from build123d import *

# Parameters (mm, degrees)
EXTRUDE064_DEPTH           = 5
EXTRUDE066_DEPTH           = 5
EXTRUDE066_PLACEMENT_ANGLE = 180
EXTRUDE065_DEPTH           = 2
EXTRUDE065_PLACEMENT_ANGLE = 180
EXTRUDE061_DEPTH           = 2
EXTRUDE063_DEPTH           = 3
EXTRUDE060_DEPTH           = 10
EXTRUDE057_DEPTH           = 5


with BuildPart() as extrude064:
    # Sketch039 → Extrude064 (new body)
    with BuildSketch(Plane.XY):
        Polygon((-0.523418, -66.073971), (-3.588769, -58.006004), (-3.588769, -66.073971), align=None)
    extrude(amount=EXTRUDE064_DEPTH)


with BuildPart() as extrude064_1:
    # Extrude064 placement: moved
    add(extrude064.part.moved(Location((-2, 0, -1))))


with BuildPart() as fusion056:
    # Sketch039 → Extrude066 (new body)
    with BuildSketch(Plane.XY):
        Polygon((-0.523418, -66.073971), (-3.588769, -58.006004), (-3.588769, -66.073971), align=None)
    extrude(amount=EXTRUDE066_DEPTH)


with BuildPart() as fusion056_1:
    # Extrude066 placement: moved
    add(fusion056.part.moved(Location((-2, -63.2, 3.5))).rotate(Axis((-2, -63.2, 3.5), (1, 0, 0)), EXTRUDE066_PLACEMENT_ANGLE))

    # Fusion056: union Extrude064
    add(extrude064_1.part)


with BuildPart() as extrude065:
    # Sketch037 → Extrude065 (new body)
    with BuildSketch(Plane.XY):
        Polygon((-0.523418, -66.073971), (-3.588769, -58.006004), (-3.588769, -66.073971), align=None)
    extrude(amount=EXTRUDE065_DEPTH)


with BuildPart() as extrude065_1:
    # Extrude065 placement: moved
    add(extrude065.part.moved(Location((-0.5, -63.2, 2.45))).rotate(Axis((-0.5, -63.2, 2.45), (1, 0, 0)), EXTRUDE065_PLACEMENT_ANGLE))


with BuildPart() as fusion055:
    # Sketch037 → Extrude061 (new body)
    with BuildSketch(Plane.XY):
        Polygon((-0.523418, -66.073971), (-3.588769, -58.006004), (-3.588769, -66.073971), align=None)
    extrude(amount=EXTRUDE061_DEPTH)


with BuildPart() as fusion055_1:
    # Extrude061 placement: moved
    add(fusion055.part.moved(Location((-0.5, 0, 0.4))))

    # Fusion055: union Extrude065
    add(extrude065_1.part)


with BuildPart() as extrude063:
    # Sketch038 → Extrude063 (new body)
    with BuildSketch(Plane.YZ):
        with BuildLine():
            ThreePointArc((-52.009312, -0.734582), (-31.50638, -4.580156), (-11.018523, -0.655055))
            ThreePointArc((-5.240026, 0.419738), (-8.178332, 0.146093), (-11.018523, -0.655055))
            Line((-5.240026, 0.419738), (2.759974, 0.419738))
            Line((2.759974, 0.419738), (2.759974, 2.419738))
            Line((2.759974, 2.419738), (-5.240026, 2.419738))
            ThreePointArc((-5.240026, 2.419738), (-8.772288, 2.061286), (-12.172965, 1.041109))
            ThreePointArc((-51.872542, 1.363439), (-32.05345, -2.578482), (-12.172965, 1.041109))
            ThreePointArc((-51.872542, 1.363439), (-54.88716, 2.147131), (-57.990026, 2.419738))
            Line((-65.990026, 2.419738), (-57.990026, 2.419738))
            Line((-65.990026, 0.419738), (-65.990026, 2.419738))
            Line((-57.990026, 0.419738), (-65.990026, 0.419738))
            ThreePointArc((-52.009312, -0.734582), (-54.946975, 0.115595), (-57.990026, 0.419738))
        make_face()
    extrude(amount=EXTRUDE063_DEPTH)


with BuildPart() as extrude063_1:
    # Extrude063 placement: moved
    add(extrude063.part.moved(Location((-7, 0, 0))))


with BuildPart() as extrude060:
    # Sketch036 → Extrude060 (new body)
    with BuildSketch(Plane.XY):
        Polygon((-0.489114, -59.765606), (-2.785057, -58.065606), (-2.989114, -56.006916), (-2.989114, -7.606139), (-2.772346, -5.215606), (-0.489114, -3.515606), align=None)
    extrude(amount=EXTRUDE060_DEPTH)


with BuildPart() as extrude060_1:
    # Extrude060 placement: moved
    add(extrude060.part.moved(Location((0, 0, -6))))


with BuildPart() as obj1:
    # Sketch033 → Extrude057 (new body)
    with BuildSketch(Plane.YZ):
        with BuildLine():
            ThreePointArc((-52.506138, -1.600172), (-31.607264, -5.496793), (-10.720935, -1.533483))
            ThreePointArc((-5.324033, -0.496866), (-8.066716, -0.784889), (-10.720935, -1.533483))
            Line((-5.324033, -0.496866), (2.675967, -0.496866))
            Line((2.675967, -0.496866), (2.675967, 3.003134))
            Line((2.675967, 3.003134), (-5.324033, 3.003134))
            ThreePointArc((-5.324033, 3.003134), (-8.649812, 2.668233), (-11.870907, 1.7752))
            ThreePointArc((-52.088632, 2.000492), (-32.001526, -1.996019), (-11.870907, 1.7752))
            ThreePointArc((-52.088632, 2.000492), (-55.042543, 2.733373), (-58.074033, 3.003134))
            Line((-66.074033, 3.003134), (-58.074033, 3.003134))
            Line((-66.074033, -0.496866), (-66.074033, 3.003134))
            Line((-58.074033, -0.496866), (-66.074033, -0.496866))
            ThreePointArc((-52.506138, -1.600172), (-55.241791, -0.804798), (-58.074033, -0.496866))
        make_face()
    extrude(amount=EXTRUDE057_DEPTH)


with BuildPart() as obj1_1:
    # Extrude057 placement: moved
    add(obj1.part.moved(Location((-5.5, 0.1, 0.15))))

    # Cut060: cut Extrude060
    add(extrude060_1.part, mode=Mode.SUBTRACT)

    # Cut061: cut Extrude063
    add(extrude063_1.part, mode=Mode.SUBTRACT)

    # Cut062: cut Fusion055
    add(fusion055_1.part, mode=Mode.SUBTRACT)

    # Cut063: cut Fusion056
    add(fusion056_1.part, mode=Mode.SUBTRACT)


with BuildPart() as obj1_2:
    # Cut063 placement: moved
    add(obj1_1.part.moved(Location((0, 0, -0.15))))


solid = obj1_2.part
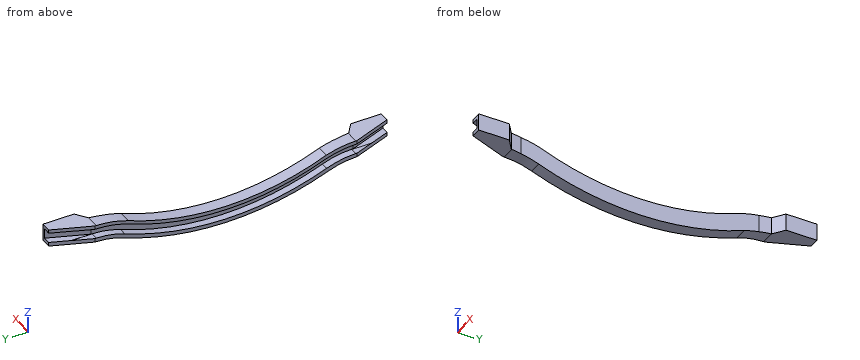
The model under review builds one solid part; all positions refer to its coordinate system, in mm. Coordinates: 2 decimals unless noted, no trailing zeros. Write each loop counter-clockwise with the first axis right and the second up, starting at its lowest first coordinate (ties: lowest second). Pieces come first, ordered by that corner, then holes. Notation, with made-up numbers: M 22.5,-30 L 75.5,-30 A13 cw 75.5,-11 Z; hole C 55,-35.75 d8. An arc over 180 degrees is marked long. Put each result on its own line as item: value.
1) Clearance check with flat-ended pins moving along their axes: pin 1 Ø2 at (x, y) = (-4.5, -44.5) entering from -Z; pin 2 Ø2.5 at (x, y) = (-3.5, -60.5) entering from -Z. State where each tip first meets the part, or that it passes through.
Computed:
pin 1: stops at z = -4.25
pin 2: stops at z = -0.5
2) Add section A-A on y = -33.5. Give the boundary of the cut face in (x, z).
Computed:
outline: M -5.5,-5.47 L -2.99,-5.47 L -2.99,-1.96 L -5.5,-1.96 L -5.5,-2.7 L -4,-2.7 L -4,-4.7 L -5.5,-4.7 Z
3) Add section B-B on y = -21.5. Give the boundary of the cut face in (x, z).
Computed:
outline: M -5.5,-4.6 L -2.99,-4.6 L -2.99,-1.04 L -5.5,-1.04 L -5.5,-1.77 L -4,-1.77 L -4,-3.81 L -5.5,-3.81 Z
4) Wall thickness on probe 1 along Z at (x, y) = (-3.9, -61); probe 2 along X at (y, z) = (-21.5, -3.75); probe 3 along Z at (x, y) = (-4.6, -36.5): over which ranges is each line inside the solid? List them lowest first. Write a range as [from, to].
Computed:
probe 1: z = [-0.5, 0.25], [2.25, 3]
probe 2: x = [-4, -2.99]
probe 3: z = [-5.29, -4.52], [-2.51, -1.77]
